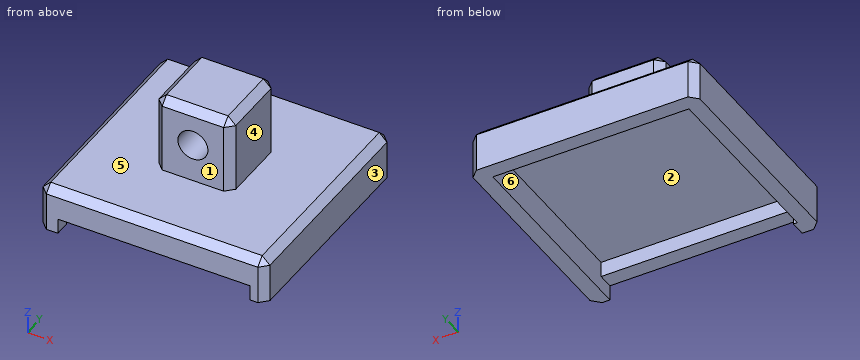
Autodesk Inventor part; units mm, degrees
ref_plane "YZ Plane" through (0, 0, 0) normal (1, 0, 0) x (0, 1, 0)
ref_plane "XZ Plane" through (0, 0, 0) normal (0, 1, 0) x (-1, 0, 0)
ref_plane "XY Plane" through (0, 0, 0) normal (0, 0, 1) x (1, 0, 0)
sketch "Skizze1" plane through (0, 0, 0) normal (0, 0, 1) x (1, 0, 0)
  point P0 (0, 0)
sketch "Skizze2" plane through (0, 0, 0) normal (0, 0, 1) x (1, 0, 0)
  line L0 (-12.75, 12.25) -> (12.75, 12.25)
  line L1 (12.75, 12.25) -> (12.75, -12.25)
  line L2 (12.75, -12.25) -> (-12.75, -12.25)
  line L3 (-12.75, -12.25) -> (-12.75, 12.25)
  line L4 (0, 19.95) -> (0, -19.95)
  line L5 (-20.65, 0) -> (20.65, 0)
  line L6 (-14.75, 14.25) -> (14.75, 14.25)
  line L7 (14.75, 14.25) -> (14.75, -14.25)
  line L8 (14.75, -14.25) -> (-14.75, -14.25)
  line L9 (-14.75, -14.25) -> (-14.75, 14.25)
  point P0 (0, 0)
  dimension "d0" = 25.5
  dimension "d1" = 24.5
  dimension "d2" = 2
  dimension "d3" = 2
  dimension "d4" = 2
  dimension "d5" = 2
extrude "Extrusion1" add sketch "Skizze2" along normal blind 4 contours L3 L5 L9 L6 L4 L0 | L4 L6 L7 L5 L1 L0 | L3 L2 L4 L8 L9 L5 | L5 L7 L8 L4 L2 L1
sketch "Skizze3" plane through (0, 0, 4) normal (0, 0, 1) x (1, 0, 0)
  line L0 (14.75, -14.25) -> (-14.75, -14.25)
  line L1 (-14.75, 14.25) -> (14.75, 14.25)
  line L2 (14.75, 14.25) -> (14.75, -14.25)
  line L3 (14.75, -14.25) -> (-14.75, -14.25)
  line L4 (-14.75, -14.25) -> (-14.75, 14.25)
  point P0 (0, 0)
extrude "Extrusion2" add sketch "Skizze3" along normal blind 2
chamfer "Fase1" distance 1 angle 45 8 edges at (14.75, 14.25, 3) (-14.75, 14.25, 3) (-14.75, 0, 6) (0, -14.25, 6) (-14.75, -14.25, 3) (14.75, -14.25, 3) (14.75, 0, 6) (0, 14.25, 6)
sketch "Skizze4" plane through (0, 0, 0) normal (0, 0, -1) x (-1, 0, 0)
  line L0 (12.75, -12.25) -> (-12.75, -12.25)
  line L1 (-12.75, -12.25) -> (12.25, -12.25)
  line L2 (12.25, -12.25) -> (12.25, -17.2138)
  line L3 (12.25, -17.2138) -> (-12.75, -17.2138)
  line L4 (-12.75, -17.2138) -> (-12.75, -12.25)
  point P0 (0, 0)
extrude "Extrusion3" cut sketch "Skizze4" against normal blind 2
sketch "Skizze5" plane through (0, 0, 0) normal (0, 0, -1) x (-1, 0, 0)
  circle A0 centre (0.25, 13.25) radius 0.5
  line L0 (13.75, 14.25) -> (-13.75, 14.25)
  line L1 (14.75, -13.25) -> (14.75, 13.25)
  line L2 (-14.75, 13.25) -> (-14.75, -13.25)
  circle A1 centre (-9.75, 13.25) radius 0.5
  circle A2 centre (10.25, 13.25) radius 0.5
  circle A3 centre (-13.75, 0.25) radius 0.5
  circle A4 centre (-13.75, -9.75) radius 0.5
  circle A5 centre (-13.75, 10.25) radius 0.5
  line L3 (0, -19.95) -> (0, 19.95)
  circle A6 centre (13.75, 0.25) radius 0.5
  circle A7 centre (13.75, -9.75) radius 0.5
  circle A8 centre (13.75, 10.25) radius 0.5
  point P0 (0, 0)
  dimension "d15" = 1
  dimension "d16" = 1
  dimension "d17" = 1
  dimension "d18" = 1
  dimension "d19" = 10
  dimension "d20" = 10
  dimension "d21" = 1
  dimension "d22" = 1
  dimension "d23" = 1
  dimension "d24" = 1
  dimension "d25" = 10
  dimension "d26" = 10
sketch "Skizze6" plane through (0, 0, 6) normal (0, 0, 1) x (1, 0, 0)
  line L0 (-5, 5) -> (5, 5)
  line L1 (5, 5) -> (5, -5)
  line L2 (5, -5) -> (-5, -5)
  line L3 (-5, -5) -> (-5, 5)
  line L4 (0, 19.95) -> (0, -19.95)
  line L5 (-20.65, 0) -> (20.65, 0)
  point P0 (0, 0)
  dimension "d29" = 10
  dimension "d30" = 10
extrude "Extrusion5" add sketch "Skizze6" along normal blind 10
sketch "Skizze9" plane through (-5, 5, 6) normal (0, 1, 0) x (1, 0, 0)
  circle A0 centre (5, -5) radius 1.95
  line L0 (10, -10) -> (0, -10)
  point P0 (5, 6)
  dimension "d52" = 3.9
  dimension "d53" = 5
extrude "Extrusion8" cut sketch "Skizze9" against normal blind 26
chamfer "Fase4" distance 1 angle 45 8 edges at (-5, 0, 16) (0, -5, 16) (5, -5, 11) (5, 5, 11) (0, 5, 16) (-5, 5, 11) (-5, -5, 11) (5, 0, 16)
properties part number "Raspberrycamhalter"
Here's how the part is built. I have some questions about the finished solid (model axes, mm). Face numbers are marked on the shaded views. A direction names the side the tool comes from. Give positions to 0.01 mm unless a question says otherwise; leave off trailing zeros. Order: outer loops, then holes, each group sorted by start corner. A loop starts at its lowest first (then second) coordinate and runs counter-clockwise, first axis right, second up. Notation, with made-up numbers: (87, 86) - (139, 86) arc R22 cw to (139, 110) - close; hole circle Ø6 at (68, 19). An arc over 180 degrees is marked (long way). Answer as a JSON object with one key per item and string values. Group by question number.
Item 1: For P1, Ø2, axis at y = -1.5, z = 12.5, coming from the +X side; P2, Ø1, axis at x = -1.5, y = -13, coming from the -Z side; P3, Ø5, axis at x = 0, z = 11, coming from the -Y side, each with a flat end and sliding along its axis, tell me the tip position at first contact or that it passes through.
Item 2: If we section it at B-B on y = -1: Please give me the cut outline in (x, z), and give its area (3 significant figures).
Item 3: Which directions (+Z, -Z, +X, -X, +Y, -Y) give clear straight access to the entire face, cutting with the end or side of a thin tool? Please do the marked faces 4, 5 and 6.
Item 4: If we section it at D-D on z = 3.5: Please give me the cut outline in (x, y).
Item 5: If we section it at C-C on z = 11: Please give me the cut outline in (x, y).
Item 6: If we mould it in two halves opening along X, with no side actions, what happens to the marked faces 1, 2 and 3? For each: pulls with the +X half, pulls with the -X half, needs draft (parallel to the pull), parting line crosses it, or undercut.
Item 7: If we section it at A-A on x = 0: Please give me the cut outline in (y, z).
Item 8: Please list where these lines run through material, in increasing order: probe 1 along Z at (x, y) = (0, 1.75); probe 2 along Y at (x, z) = (12.25, 2.75); probe 3 along X at (y, z) = (-2.5, 11).
Result set:
{
 "1": {"P1": "x = 5", "P2": "z = 2", "P3": "y = -5"},
 "2": {"outline": "(-14.75, 0) - (-12.75, 0) - (-12.75, 4) - (12.75, 4) - (12.75, 0) - (14.75, 0) - (14.75, 5) - (13.75, 6) - (5, 6) - (5, 15) - (4, 16) - (-4, 16) - (-5, 15) - (-5, 6) - (-13.75, 6) - (-14.75, 5) - close; hole circle Ø3.9 at (0, 11)", "area": "161 mm²"},
 "3": {"face 4": "+Z, +X, +Y, -Y", "face 5": "+Z", "face 6": "-Z"},
 "4": {"outline": "(-14.75, -13.25) - (-13.75, -14.25) - (13.75, -14.25) - (14.75, -13.25) - (14.75, 13.25) - (13.75, 14.25) - (-13.75, 14.25) - (-14.75, 13.25) - close; hole (-12.75, -12.25) - (12.75, -12.25) - (12.75, 12.25) - (-12.75, 12.25) - close"},
 "5": {"outline": "(-5, -4) - (-4, -5) - (-1.95, -5) - (-1.95, 5) - (-4, 5) - (-5, 4) - close; (1.95, -5) - (4, -5) - (5, -4) - (5, 4) - (4, 5) - (1.95, 5) - close"},
 "6": {"face 1": "needs draft", "face 2": "undercut", "face 3": "pulls with the +X half"},
 "7": {"outline": "(-14.25, 2) - (-12.25, 2) - (-12.25, 4) - (12.25, 4) - (12.25, 0) - (14.25, 0) - (14.25, 5) - (13.25, 6) - (5, 6) - (5, 9.05) - (-5, 9.05) - (-5, 6) - (-13.25, 6) - (-14.25, 5) - close; (-5, 12.95) - (5, 12.95) - (5, 15) - (4, 16) - (-4, 16) - (-5, 15) - close"},
 "8": {"probe 1": "4 to 9.05, 12.95 to 16", "probe 2": "-14.25 to -12.25, 12.25 to 14.25", "probe 3": "-5 to -1.95, 1.95 to 5"}
}
